from build123d import *

# Parameters (mm, degrees)
SKETCH_1_R          = 2
EXTRUDE_1_DEPTH     = 3
SKETCH_2_R          = 1.5
CUT_EXTRUDE_1_DEPTH = 306.548310575
FILLET_1_R          = 15
FILLET_2_R          = 5
FILLET_3_R          = 10


with BuildPart() as part:
    # 草图1 → 凸台-拉伸1 (new body)
    with BuildSketch(Plane.XY):
        Polygon((0, 0), (36, 0), (36, 28.269869579), (0, 76.702645079), (0, 226.702645079), (34.436828012, 273.032399523), (34.436828012, 303.405290157), (16.23224311, 303.405290157), (-15, 256), (-15, 26), (-9, 0), align=None)
        with Locations((26, 10)):
            Circle(SKETCH_1_R, mode=Mode.SUBTRACT)
        with Locations(Location((14.436828012, 287.405290157, 0), (0, 0, 180))):
            Circle(SKETCH_1_R, mode=Mode.SUBTRACT)
        with Locations((-2, 10)):
            Circle(SKETCH_1_R, mode=Mode.SUBTRACT)
    extrude(amount=EXTRUDE_1_DEPTH)

    # 草图2 → 切除-拉伸1 (cut, through all)
    with BuildSketch(Plane.XY.offset(3)):
        with Locations((-12, 246)):
            Circle(SKETCH_2_R)
        with Locations((-12, 221)):
            Circle(SKETCH_2_R)
        with Locations((-12, 196)):
            Circle(SKETCH_2_R)
        with Locations((-12, 171)):
            Circle(SKETCH_2_R)
        with Locations((-12, 146)):
            Circle(SKETCH_2_R)
        with Locations((-12, 121)):
            Circle(SKETCH_2_R)
        with Locations((-12, 96)):
            Circle(SKETCH_2_R)
        with Locations((-12, 71)):
            Circle(SKETCH_2_R)
    extrude(amount=-CUT_EXTRUDE_1_DEPTH, mode=Mode.SUBTRACT)

    # 圆角1
    fillet_1_edges = [part.edges().sort_by_distance(p)[0] for p in [
        (-9, 0, 1.5),
        (36, 0, 1.5),
    ]]
    fillet(fillet_1_edges, radius=FILLET_1_R)

    # 圆角2
    fillet_2_edges = [part.edges().sort_by_distance(p)[0] for p in [
        (-15, 26, 1.5),
        (-15, 256, 1.5),
        (16.23224311, 303.405290157, 1.5),
        (34.436828012, 273.032399523, 1.5),
        (0, 226.702645079, 1.5),
        (0, 76.702645079, 1.5),
        (36, 28.269869579, 1.5),
    ]]
    fillet(fillet_2_edges, radius=FILLET_2_R)

    # 圆角3
    fillet_3_edges = [part.edges().sort_by_distance(p)[0] for p in [
        (34.436828012, 303.405290157, 1.5),
    ]]
    fillet(fillet_3_edges, radius=FILLET_3_R)


solid = part.part
Verification items for the finished model (mm, model axes). A direction names the side the tool comes from. Coordinates: 2 decimals unless noted, no trailing zeros. Order: outer loops, then holes, each group sorted by start corner. A loop starts at its lowest first (then second) coordinate and runs counter-clockwise, first axis right, second up. Notation, with made-up numbers: M 77,60 L 83,60 A15 ccw 83,70 Z; hole C -40,-23.5 d1. An arc over 180 degrees is marked long. Return JSON: item names as keys, results as strings.
1) Access from +Z, -Z, +X, -X, +Y, -Y to the whole of each face (thin tool, end or side, straight path). Record for faces 1 (the flat face through (-1, 120, 3)), 2 (the flat face through (16.99, 249.56, 1.48)).
Answer list:
{"face 1": "+Z, +X, -X, +Y, -Y", "face 2": "+Z, -Z, +X"}
2) Thickness scan on L1, parallel to X at y = 146, z = 1.45; L2, parallel to X at y = 176, z = 1.7; L3, parallel to Y at x = 9.5, z = 1.55. Record the ranges inside material, lowest first. Write a range as [from, to].
Answer list:
{"L1": "[-15, -13.5], [-10.5, 0]", "L2": "[-15, 0]", "L3": "[0, 63.92], [239.48, 293.19]"}
3) Cross-section at B-B, the plane y = 110. Record the boundary of the cut face in (x, z), and give its area (3 significant figures).
Answer list:
{"outline": "M -15,0 L 0,0 L 0,3 L -15,3 Z", "area": "45.0 mm2"}
4) Cross-section at A-A, the plane z = 0.85. Count the separate pieces of the cut face and the enclosed holes in it, and give its area (3 significant figures).
Answer list:
{"separate pieces": "1", "enclosed holes": "11", "area": "7,270 mm2"}
5) Release check for a two-part mould opening along Y. For faces 3 (the cylindrical face through (31.585, 300.398, 1.521)), 4 (the cylindrical face through (31.72, 4.51, 1.52)), 5 (the flat face through (-1, 120, 0)), 6 (the flat face through (18.238, 52.166, 1.479)) record: +Y half, -Y half, draft (parallel to the pull), parting line (faces both ways), or undercut.
Answer list:
{"face 3": "+Y half", "face 4": "-Y half", "face 5": "draft", "face 6": "undercut"}
6) Cross-section at C-C, the plane x = -7. Record the boundary of the cut face in (y, z).
Answer list:
{"outline": "M 3.76,0 L 268.14,0 L 268.14,3 L 3.76,3 Z"}
